Input: dimensioned drawing with shaded views. Units: mm. Origin: part minimum x, y, z. Round coordinates to 2 decimals unless told otherwise and drop trailing zeros. Loops run counter-clockwise (first coordinate to the right, second up) from the corner with the lowest first, then second, coordinate; pieces in that order, holes last. Notation, with made-up numbers: M 82.5,10 L 122.5,10 A12 cw 122.5,30 Z; hole C 83,87.5 d6. An arc over 180 degrees is marked long. Write each question's results on one line, items separated by ' | '. Start each with the question number.
1. Ray query, line 1 (X direction, y = 0.95, z = 25.5); line 2 (Z direction, x = 3.85, y = 0.85). Return the intervals inside material, ascending.
2. Contact query for a flat-ended pin moving along its axis: pin 1 Ø4.5 at (x, z) = (77.45, 25.5) entering from +Y. Output: stop coordinate, or through.
3. Section A-A on x = 3.85. Output: boundary loops of the cut face in (y, z), and give its area (4 significant figures).
4. Section B-B on z = 25.5. Output: boundary loops of the cut face in (x, y).
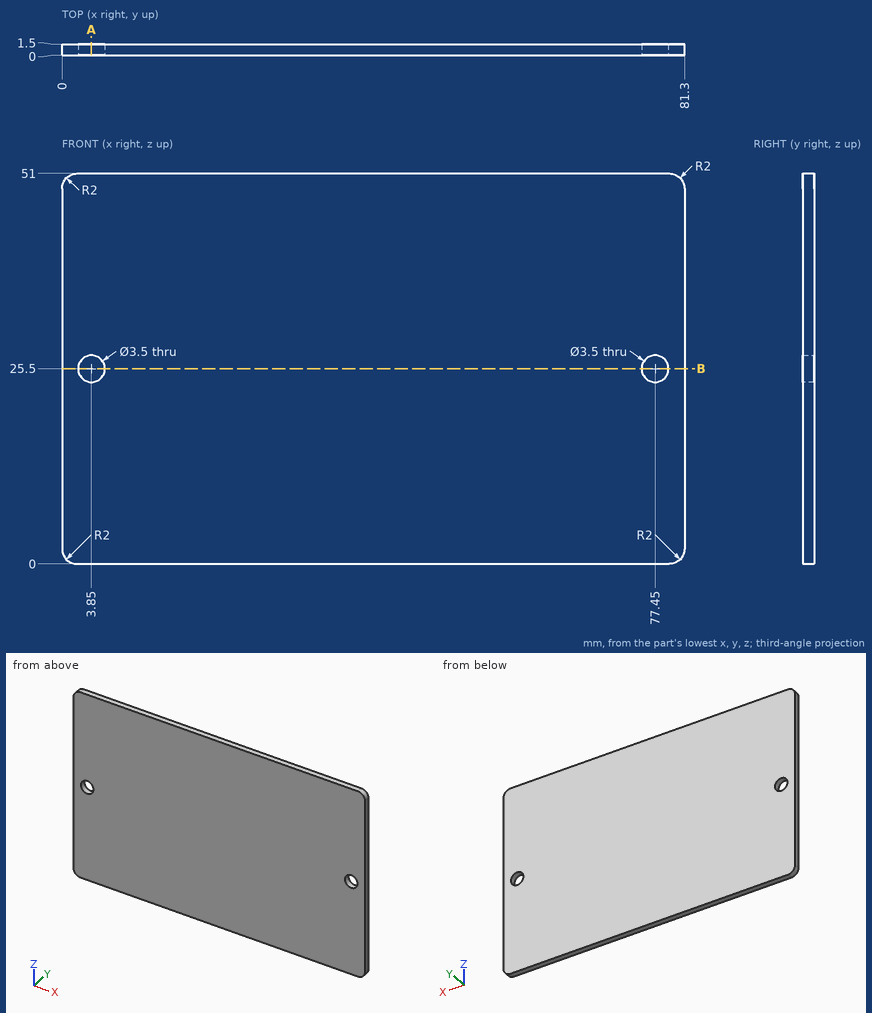
Taken from the geometry:
1) line 1: 0 to 2.1, 5.6 to 75.7, 79.2 to 81.3 | line 2: 0 to 23.75, 27.25 to 51
2) pin 1: y = 1.5
3) outline: M 0,0 L 1.5,0 L 1.5,23.75 L 0,23.75 Z; M 0,27.25 L 1.5,27.25 L 1.5,51 L 0,51 Z | area: 71.25 mm^2
4) outline: M 0,0 L 2.1,0 L 2.1,1.5 L 0,1.5 Z; M 5.6,0 L 75.7,0 L 75.7,1.5 L 5.6,1.5 Z; M 79.2,0 L 81.3,0 L 81.3,1.5 L 79.2,1.5 Z
